Could you check a few things on this model? Use its own coordinates, in mm. Give positions to 0.01 mm unless a question says otherwise; leave off trailing zeros. Loops run counter-clockwise (first coordinate to the right, second up) from the corner with the lowest first, then second, coordinate; pieces in that order, holes last.
1. Imagine slicing it at C-C (x = 0). Count the separate pieces of the cut face and the enclosed holes in it, plus the area to 3 significant figures.
2. Imagine slicing it at A-A (y = -22). List the corners of the cut face in (x, z) for me.
3. Imagine slicing it at B-B (z = 6.5). List the corners of the cut face in (x, y) for me.
4. Thinking about a two-plate mould opening in Y: for faces 1 (the flat face through (-15, -17.7, 7.9)), 2 (the cylindrical face through (10.23, 6.2, 6.41)), 3 (the cylindrical face through (-27.409, 13.105, 6.584)), which applies, +Y half, -Y half, draft (parallel to the pull), parting line (faces both ways), or undercut?
5. For P1, Ø9.5, axis at x = -29.35, y = 16.83, coming from the +Z side; P2, Ø4, axis at y = -18, z = 8, coming from the -X side, each with a flat end and sliding along its axis, tell me the tip position at first contact or that it passes through.
6. I need wall thicknesses on line 1 along Y through (x, z) = (-0.5, 5.5); line 2 along Y through (x, z) = (-3.5, 4.75); line 3 along Y through (x, z) = (-5.5, 6.75). Which ranges of each line are inside material? Lowest first, please.
```python
from build123d import *

# Parameters (mm, degrees)
BOSS_EXTRUDE1_DEPTH        = 13
CUT_EXTRUDE1_DEPTH         = 55.223360011
CUT_EXTRUDE2_DEPTH         = 55.01851513
F_8_4_8_4_DIAMETER_HOLE1_D = 8.4
CHAMFER2_SIZE              = 0.5


with BuildPart() as part:
    # Sketch1 → Boss-Extrude1 (new body)
    with BuildSketch(Plane(origin=(0, 0, 0), x_dir=(-1, 0, 0), z_dir=(0, 0, -1))):
        with BuildLine():
            Line((-14.999999535, -11.339745693), (-14.999999535, -27.999999731))
            ThreePointArc((-14.999999535, -27.999999731), (4.65e-07, -42.999999731), (15.000000465, -27.999999731))
            Line((15.000000465, -27.999999731), (15.000000465, -13.660253769))
            ThreePointArc((15.000000465, -13.660253769), (16.160254503, -9.33012675), (19.330127484, -6.160253769))
            Line((19.330127484, -6.160253769), (31.748711306, 1.009618943))
            ThreePointArc((31.748711306, 1.009618943), (37.239092363, 6.5), (39.248711306, 14))
            ThreePointArc((39.248711306, 14), (37.239092363, 21.5), (31.748711306, 26.990381057))
            ThreePointArc((31.748711306, 26.990381057), (24.248711306, 29), (16.748711306, 26.990381057))
            Line((16.748711306, 26.990381057), (2.320508541, 18.660254307))
            ThreePointArc((2.320508541, 18.660254307), (-10.358983383, 5.980762382), (-14.999999535, -11.339745693))
        make_face()
    extrude(amount=-BOSS_EXTRUDE1_DEPTH)

    # Sketch2 → Cut-Extrude1 (cut, through all)
    with BuildSketch(Plane(origin=(-7.5, -12.990381057, 0), x_dir=(0.8660254037844388, -0.4999999999999997, 0), z_dir=(-0.4999999999999997, -0.8660254037844388, 0))):
        with BuildLine():
            ThreePointArc((-25.021227161, 9.417565156), (-22, 2.3), (-18.978772839, 9.417565156))
            ThreePointArc((-18.978772839, 9.417565156), (-22, 10.7), (-25.021227161, 9.417565156))
        make_face()
    extrude(amount=-CUT_EXTRUDE1_DEPTH, mode=Mode.SUBTRACT)

    # Sketch3 → Cut-Extrude2 (cut, through all)
    with BuildSketch(Plane.ZY.offset(15.000000465)):
        with BuildLine():
            ThreePointArc((9.417565156, -18.978772839), (2.3, -22), (9.417565156, -25.021227161))
            ThreePointArc((9.417565156, -25.021227161), (10.7, -22), (9.417565156, -18.978772839))
        make_face()
    extrude(amount=-CUT_EXTRUDE2_DEPTH, mode=Mode.SUBTRACT)

    # Ø8.4 (8.4) Diameter Hole1 (through all)
    with Locations(Plane(origin=(0, 0, 0), x_dir=(-1, 0, 0), z_dir=(0, 0, -1))):
        with Locations((29.347432097, 16.831243464), (0.097432097, -33.831242658)):
            Hole(F_8_4_8_4_DIAMETER_HOLE1_D / 2)

    # Chamfer2
    chamfer2_edges = [part.edges().sort_by_distance(p)[0] for p in [
        (-4.297432097, -33.831242658, 0),
        (-4.297432097, -33.831242658, 13),
        (-33.547432097, 16.831243464, 0),
        (-33.547432097, 16.831243464, 13),
    ]]
    chamfer(chamfer2_edges, length=CHAMFER2_SIZE)


solid = part.part
```
Derived:
1. separate pieces: 2
1. enclosed holes: 1
1. area: 617 mm2
2. outline: (-15, 0) - (15, 0) - (15, 2.3) - (-15, 2.3) - close; (-15, 10.7) - (15, 10.7) - (15, 13) - (-15, 13) - close
3. outline: (-31.75, 1.01) - (-30.19, 0.11) - (-15.19, 26.09) - (-16.75, 26.99) arc R15 ccw to start; (-22.92, -4.09) - (-19.33, -6.16) arc R8.66 cw to (-15, -13.66) - (-15, -17.8) - (15, -17.8) - (15, -11.34) arc R34.64 ccw to (-2.32, 18.66) - (-7.92, 21.89) - close; (-15, -28) arc R15 ccw to (15, -28) - (15, -26.2) - (-15, -26.2) - close; hole circle Ø8.4 at (-29.35, 16.83); hole circle Ø8.4 at (-0.1, -33.83)
4. face 1: draft
4. face 2: +Y half
4. face 3: undercut
5. P1: stops at z = 13
5. P2: stops at x = -15
6. line 1: y = -42.99 to -38.01, -29.65 to -26.08, -17.92 to 17.53
6. line 2: y = -42.59 to -36.29, -31.37 to -25.82, -18.18 to 19.34
6. line 3: y = -41.96 to -26.19, -17.81 to 20.5
